Read the model definition and answer for the solid it produces. Units are mm, in the model's axes. A direction names the side the tool comes from. Round coordinates to 2 decimals unless told otherwise and drop trailing zeros. Loops run counter-clockwise (first coordinate to the right, second up) from the corner with the lowest first, then second, coordinate; pieces in that order, holes last. Notation, with made-up numbers: (29.25, 5.25) - (49.25, 5.25) arc R12 ccw to (49.25, 15.25) - close; hole circle Ø2 at (31, -31.75). An arc over 180 degrees is marked (long way). Answer as CSV lines item,"result".
Autodesk Inventor part; units mm, degrees
ref_plane "YZ Plane" through (0, 0, 0) normal (1, 0, 0) x (0, 1, 0)
ref_plane "XZ Plane" through (0, 0, 0) normal (0, 1, 0) x (-1, 0, 0)
ref_plane "XY Plane" through (0, 0, 0) normal (0, 0, 1) x (1, 0, 0)
sketch "Sketch1" plane through (0, 0, 0) normal (0, 1, 0) x (-1, 0, 0)
  line L0 (0, 0) -> (48.3455, 0)
  line L1 (48.3455, 0) -> (48.3455, -113.25)
  line L2 (48.3455, -113.25) -> (0, -113.25)
  line L3 (0, -113.25) -> (0, 0)
  line L4 (27.1728, 0) -> (21.1727, 0)
  line L5 (21.1727, 0) -> (21.1727, -21.95)
  line L6 (21.1727, -21.95) -> (27.1728, -21.95)
  line L7 (27.1728, -21.95) -> (27.1728, 0)
  line L8 (29.1728, 0) -> (19.1728, 0)
  line L9 (19.1728, 0) -> (19.1728, -3.302)
  line L10 (19.1728, -3.302) -> (29.1728, -3.302)
  line L11 (29.1728, -3.302) -> (29.1728, 0)
  point P0 (27.1728, -3.302)
  point P1 (21.1727, -3.302)
  dimension "d0" = 113.25
  dimension "d1" = 48.3455
  dimension "d2" = 91.3
  dimension "d3" = 6
  dimension "d4" = 21.1728
  dimension "d5" = 21.1728
  dimension "d6" = 10
  dimension "d7" = 3.302
  dimension "d8" = 2
  dimension "d9" = 2
extrude "Extrusion1" add sketch "Sketch1" along normal mid plane 3 contours L0 L9 L10 L5 L6 L7 L11 L1 L2 L3
sketch "Sketch2" plane through (0, 1.5, 0) normal (0, 1, 0) x (1, 0, 0)
  line L0 (-48.3455, 0) -> (-29.1728, 0)
  line L1 (-32.4278, 0) -> (-15.9178, 0)
  line L2 (-15.9178, 0) -> (-24.1728, 9.721)
  line L3 (-24.1728, 9.721) -> (-32.4278, 0)
  line L4 (-29.1728, 0) -> (-29.1728, 3.302)
  line L5 (-19.1728, 3.302) -> (-19.1728, 0)
  point P0 (0, 0)
  dimension "d12" = 8.255
  dimension "d13" = 16.51
  dimension "d14" = 8.255
  dimension "d15" = 3.255
  dimension "d16" = 3.255
extrude "Extrusion2" cut sketch "Sketch2" against normal up to surface (3 mm away)
fillet "Fillet1" radius 3.175 4 edges at (-27.1728, 0, -6.1882) (-21.1728, 0, -6.1882) (-32.4278, 0, 0) (-15.9178, 0, 0)
equation "\"d4\" = d5"
equation "\"d8\" = d9"
equation "\"d12\" = d14"
equation "\"d15\" = d16"
properties part number "avbay sled"
1) The mould has two halves that part along X. Classify faces 1 (the face through (0, 0, -57)), 2 (the face through (-7, 0, 0)), 3 (the face through (-15.8, 0, -0.3)): pulls with the +X half, pulls with the -X half, needs draft (parallel to the pull), parting line crosses it, or undercut.
Entries:
face 1,"pulls with the +X half"
face 2,"needs draft"
face 3,"undercut"
2) A cutting plane is placed at A-A, the plane z = -14. Determine the outline of the cut face in (x, y), plus the area to 3 significant figures.
Entries:
outline,"(-48.35, -1.5) - (-27.17, -1.5) - (-27.17, 1.5) - (-48.35, 1.5) - close; (-21.17, -1.5) - (0, -1.5) - (0, 1.5) - (-21.17, 1.5) - close"
area,"127 mm^2"
3) A cutting plane is placed at C-C, the plane x = -24.5. Determine the outline of the cut face in (y, z), plus the area to 3 significant figures.
Entries:
outline,"(-1.5, -113.25) - (1.5, -113.25) - (1.5, -21.95) - (-1.5, -21.95) - close"
area,"274 mm^2"
4) Find the intervals of material crossed by line 1 (X direction, y = -0.95, z = -15); line 2 (Z direction, x = -23, y = 0.3); line 3 (Z direction, x = -27.5, y = 1.2), in increasing order.
Entries:
line 1,"x = -48.35 to -27.17, -21.17 to 0"
line 2,"z = -113.25 to -21.95"
line 3,"z = -113.25 to -5.95"
5) A tool of negligible diameter and unlimited length cuts with its end or side. For faces 4 (the face through (-24, 1.5, -56)), 5 (the face through (-20.97, -0.02, -6.24)), from which of +Z, -Z, +X, -X, +Y, -Y can it reach the whole face along a straight path? Write none if from no direction.
Entries:
face 4,"+Z, -Z, +X, -X, +Y"
face 5,"+Z, +Y, -Y"
